Solid Edge part; units mm, degrees
sketch "Sketch1" plane through (0, 0, 0) normal (0, 0, 1) x (1, 0, 0)
  line L0 (0, 0) -> (0, 230)
  line L1 (0, 230) -> (236.5069, 230)
  line L2 (236.5069, 230) -> (236.5069, 0)
  line L3 (236.5069, 0) -> (0, 0)
sketch "Sketch2" plane through (0, 0, 0) normal (0, -1, 0) x (1, 0, 0)
  line L0 (0, 32.0927) -> (0, 5.0927)
  line L1 (0, 5.0927) -> (15.6, 5.0927)
  line L2 (15.6, 5.0927) -> (15.6, -5.6244)
  line L3 (15.6, -5.6244) -> (14.4, -5.6244)
  line L4 (14.4, 3.8927) -> (14.4, -5.6244)
  line L5 (-1.2, 3.8927) -> (14.4, 3.8927)
  line L6 (-1.2, 33.2927) -> (-1.2, 3.8927)
  line L7 (18.5085, 33.2927) -> (-1.2, 33.2927)
  line L8 (18.5085, 33.2927) -> (18.5085, 32.0927)
  line L9 (18.5085, 32.0927) -> (0, 32.0927)
sweep "ProtrusioneScorrimento_1" add profiles "Sketch2" path "Sketch1"
Geometry check sheet. Reference: the model listing, model coordinates, mm. A direction names the side the tool comes from. Coordinates: 2 decimals unless noted, no trailing zeros. Order: outer loops, then holes, each group sorted by start corner. A loop starts at its lowest first (then second) coordinate and runs counter-clockwise, first axis right, second up. Notation, with made-up numbers: (28.5, 12.5) - (32.5, 12.5) arc R11 ccw to (32.5, 26.5) - close; hole circle Ø4 at (81.5, -13.5). An arc over 180 degrees is marked (long way). One line per item, written item: value.
(1) Depth check by flat-ended pin: pin 1 Ø3 at (x, z) = (104, 0.5) entering from -Y; pin 2 Ø8.5 at (y, z) = (153.5, 1) entering from -X; pin 3 Ø10.5 at (y, z) = (141, -3) entering from +X; pin 4 Ø8.5 at (x, z) = (78.5, -3) entering from +Y. Enter the tip coordinate at first touch or a pass-through.
Data:
pin 1: stops at y = 14.4
pin 2: stops at x = -1.2
pin 3: stops at x = 222.11
pin 4: stops at y = 215.6
(2) Access from +Z, -Z, +X, -X, +Y, -Y to the whole of each face (thin tool, end or side, straight path). Record for faces 1 (the face through (117, 14.4, -1)), 2 (the face through (220.907, 114, 0)), 3 (the face through (120, 11, 32.093)).
Data:
face 1: -Z, +X, -X, -Y
face 2: -Z
face 3: none
(3) Thickness scan on probe 1 along Y at (x, z) = (187, 27.5); probe 2 along X at (y, z) = (48.5, 19); probe 3 along Y at (x, z) = (91, -3). Record the ranges inside material, lowest first. Write a range as from..to.
Data:
probe 1: y = -1.2..0, 230..231.2
probe 2: x = -1.2..0, 236.51..237.71
probe 3: y = 14.4..15.6, 214.4..215.6
(4) Release check for a two-part mould opening along Z. For faces 4 (the face through (0, 117, 19)), 5 (the face through (120, 217, 33.293)), 6 (the face through (222.107, 114, -1)) record: +Z half, -Z half, draft (parallel to the pull), parting line (faces both ways), or undercut.
Data:
face 4: undercut
face 5: +Z half
face 6: draft
(5) Sectioned sample at B-B (x = 142.5). Enter the section's corners in (y, z), and give its area (3 significant figures).
Data:
outline: (-1.2, 3.89) - (14.4, 3.89) - (14.4, -5.62) - (15.6, -5.62) - (15.6, 5.09) - (0, 5.09) - (0, 32.09) - (18.51, 32.09) - (18.51, 33.29) - (-1.2, 33.29) - close; (211.49, 32.09) - (230, 32.09) - (230, 5.09) - (214.4, 5.09) - (214.4, -5.62) - (215.6, -5.62) - (215.6, 3.89) - (231.2, 3.89) - (231.2, 33.29) - (211.49, 33.29) - close
area: 175 mm^2
(6) Sectioned sample at C-C (z = 12.5). Enter the section's corners in (x, y).
Data:
outline: (-1.2, -1.2) - (237.71, -1.2) - (237.71, 231.2) - (-1.2, 231.2) - close; hole (0, 0) - (236.51, 0) - (236.51, 230) - (0, 230) - close
(7) Sectioned sample at A-A (y = 162). Enter the section's corners in (x, z).
Data:
outline: (-1.2, 3.89) - (14.4, 3.89) - (14.4, -5.62) - (15.6, -5.62) - (15.6, 5.09) - (0, 5.09) - (0, 32.09) - (18.51, 32.09) - (18.51, 33.29) - (-1.2, 33.29) - close; (218, 32.09) - (236.51, 32.09) - (236.51, 5.09) - (220.91, 5.09) - (220.91, -5.62) - (222.11, -5.62) - (222.11, 3.89) - (237.71, 3.89) - (237.71, 33.29) - (218, 33.29) - close
